Could you check a few things on this model? Use its own coordinates, in mm. Coordinates: 2 decimals unless noted, no trailing zeros. Loops run counter-clockwise (first coordinate to the right, second up) from the corner with the lowest first, then second, coordinate; pieces in that order, holes last.
from build123d import *

# Parameters (mm, degrees)
SKETCH2_W           = 30
SKETCH2_H           = 30
BOSS_EXTRUDE1_DEPTH = 252
SKETCH3_R           = 15
BOSS_EXTRUDE2_DEPTH = 10
SKETCH4_R           = 2.5
CUT_EXTRUDE1_DEPTH  = 4


with BuildPart() as part:
    # Sketch2 → Boss-Extrude1 (new body)
    with BuildSketch(Plane(origin=(0, 0, 0), x_dir=(0, 0, -1), z_dir=(1, 0, 0))):
        with Locations((15, 15)):
            Rectangle(SKETCH2_W, SKETCH2_H)
    extrude(amount=BOSS_EXTRUDE1_DEPTH)

    # Sketch3 → Boss-Extrude2 (add)
    with BuildSketch(Plane.XY):
        with Locations((237, 15)):
            Circle(SKETCH3_R)
    extrude(amount=BOSS_EXTRUDE2_DEPTH)

    # Sketch4 → Cut-Extrude1 (cut)
    with BuildSketch(Plane.XY.offset(10)):
        with Locations((237, 15)):
            Circle(SKETCH4_R)
    extrude(amount=-CUT_EXTRUDE1_DEPTH, mode=Mode.SUBTRACT)


solid = part.part
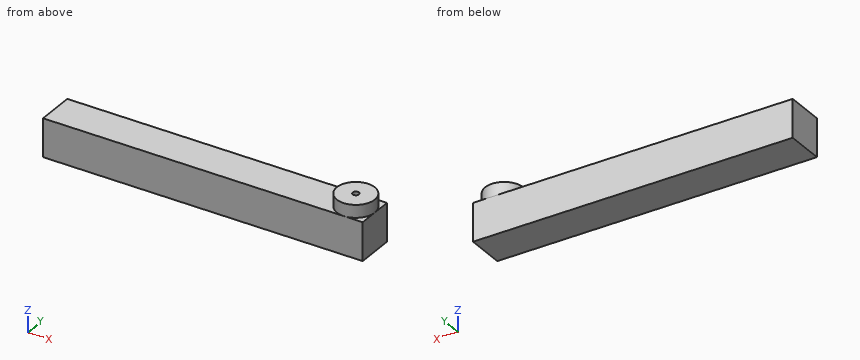
1) Imagine slicing it at A-A on y = 6.75. List the corners of the cut face in (x, z) for me, plus the area to 3 significant figures.
2) Imagine slicing it at B-B on x = 91.5. List the corners of the cut face in (y, z) for me.
3) Will these pins go through, and if not, where does the flat tip stop? pin 1 (9 mm diameter, centred on x = 101.5, y = 20, fed in from +Z); pin 2 (4 mm diameter, centred on x = 237, y = 15, fed in from +Z).
4) If I drill on L1, parallel to Y at x = 237, z = 8.95; L2, parallel to Z at x = 170, y = 10; L3, parallel to X at y = 15.75, z = 5.5, over which ranges is the centre line in solid material (lowest first)?
Solved:
1. outline: (0, -30) - (252, -30) - (252, 0) - (249.53, 0) - (249.53, 10) - (224.47, 10) - (224.47, 0) - (0, 0) - close
1. area: 7,810 mm2
2. outline: (0, -30) - (30, -30) - (30, 0) - (0, 0) - close
3. pin 1: stops at z = 0
3. pin 2: stops at z = 6
4. L1: y = 0 to 12.5, 17.5 to 30
4. L2: z = -30 to 0
4. L3: x = 222.02 to 251.98
